from build123d import *


with BuildPart() as part:
    # Skica1 → Rotovat1 (revolve)
    with BuildSketch(Plane.XY):
        Polygon((0, 3.5), (9.75, 3.5), (9.75, 4.85), (5.25, 4.85), (5.25, 5.85), (3.25, 5.85), (3.25, 4.85), (-3.25, 4.85), (-3.25, 5.85), (-5.25, 5.85), (-5.25, 4.85), (-9.75, 4.85), (-9.75, 3.5), align=None)
    revolve(axis=Axis((0, 0, 0), (1, 0, 0)))


solid = part.part
Can you work these out from the model? Positions are in its coordinate system, mm. A direction names the side the tool comes from. Coordinates: 2 decimals unless noted, no trailing zeros. Order: outer loops, then holes, each group sorted by start corner. A loop starts at its lowest first (then second) coordinate and runs counter-clockwise, first axis right, second up. Notation, with made-up numbers: (10, 50.25) -> (65, 50.25) arc R12 cw to (65, 67.25) -> close; hole circle Ø3 at (16.25, 24.5). An arc over 180 degrees is marked (long way). Use one line per item in the form item = value.
Q1. Imagine slicing it at C-C, the plane x = -7. List the corners of the cut face in (y, z) for me, then the cut area to 3 significant figures.
From the geometry:
outline = circle Ø9.7 at (0, 0); hole circle Ø7 at (0, 0)
area = 35.4 mm²
Q2. I need wall thicknesses on L1, parallel to Z at x = 0, y = 0; L2, parallel to X at y = -4.25, z = -3.75; L3, parallel to Z at x = 6.25, y = -1.25. Which ranges of each line are inside material? Lowest first, please.
From the geometry:
L1 = -4.85 to -3.5, 3.5 to 4.85
L2 = -5.25 to -3.25, 3.25 to 5.25
L3 = -4.69 to -3.27, 3.27 to 4.69
Q3. We'd pull the mould along X, two halves only. Please class faces 1 (the face through (3.25, 1, 5)), 2 (the face through (-7.531, 4.626, 1.457)), 3 (the face through (-9.75, 4, 0)), 4 (the face through (-0.046, 4.626, 1.457)): released by +X, released by -X, zero draft, split by the parting line, or undercut.
From the geometry:
face_1 = undercut
face_2 = zero draft
face_3 = released by -X
face_4 = undercut
Q4. Imagine slicing it at D-D, the plane z = 3.75. List the corners of the cut face in (x, y) for me, then the cut area to 3 significant figures.
From the geometry:
outline = (-9.75, -3.08) -> (-5.25, -3.08) -> (-5.25, -4.49) -> (-3.25, -4.49) -> (-3.25, -3.08) -> (3.25, -3.08) -> (3.25, -4.49) -> (5.25, -4.49) -> (5.25, -3.08) -> (9.75, -3.08) -> (9.75, 3.08) -> (5.25, 3.08) -> (5.25, 4.49) -> (3.25, 4.49) -> (3.25, 3.08) -> (-3.25, 3.08) -> (-3.25, 4.49) -> (-5.25, 4.49) -> (-5.25, 3.08) -> (-9.75, 3.08) -> close
area = 131 mm²
Q5. Which directions (+Z, -Z, +X, -X, +Y, -Y) give clear straight access to the entire face, cutting with the end or side of a thin tool? Please do faces 5 (the face through (-3.25, -1, 5)), 6 (the face through (-5.25, 1, 5)), 7 (the face through (7.469, 4.626, 1.457)), 8 (the face through (4.24, -1.27, -5.71)).
From the geometry:
face_5 = none
face_6 = -X
face_7 = +X
face_8 = +X, -X
Q6. Imagine slicing it at A-A, the plane y = 0. List the corners of the cut face in (x, z) for me.
From the geometry:
outline = (-9.75, -4.85) -> (-5.25, -4.85) -> (-5.25, -5.85) -> (-3.25, -5.85) -> (-3.25, -4.85) -> (3.25, -4.85) -> (3.25, -5.85) -> (5.25, -5.85) -> (5.25, -4.85) -> (9.75, -4.85) -> (9.75, -3.5) -> (-9.75, -3.5) -> close; (-9.75, 3.5) -> (9.75, 3.5) -> (9.75, 4.85) -> (5.25, 4.85) -> (5.25, 5.85) -> (3.25, 5.85) -> (3.25, 4.85) -> (-3.25, 4.85) -> (-3.25, 5.85) -> (-5.25, 5.85) -> (-5.25, 4.85) -> (-9.75, 4.85) -> close
Q7. Will these pins go through, and if not, where does the flat tip stop? P1, Ø6, axis at x = 1.5, z = 3.5, coming from the -Y side; P2, Ø4, axis at x = 3, z = -4, coming from the +Y side.
From the geometry:
P1 = -5.75
P2 = 5.49
